from build123d import *

# Parameters (mm, degrees)
SKETCH2_R                        = 15
BOSS_EXTRUDE1_DEPTH              = 20
TAP_DRILL_FOR_M18X2_5_TAP1_D     = 15.5
TAP_DRILL_FOR_M18X2_5_TAP1_DEPTH = 15
TAP_DRILL_FOR_M18X2_5_TAP1_TIP   = 4.656669797
FILLET1_R                        = 4


with BuildPart() as part:
    # Sketch2 → Boss-Extrude1 (new body)
    with BuildSketch(Plane(origin=(0, 0, 0), x_dir=(1, 0, 0), z_dir=(0, 1, 0))):
        Circle(SKETCH2_R)
    extrude(amount=BOSS_EXTRUDE1_DEPTH)

    # Tap Drill for M18x2.5 Tap1
    with Locations(Plane(origin=(0, 0, 0), x_dir=(-1, 0, 0), z_dir=(0, -1, 0))):
        with Locations((0, 0)):
            Hole(TAP_DRILL_FOR_M18X2_5_TAP1_D / 2, depth=TAP_DRILL_FOR_M18X2_5_TAP1_DEPTH)
            with Locations((0, 0, -(TAP_DRILL_FOR_M18X2_5_TAP1_DEPTH + TAP_DRILL_FOR_M18X2_5_TAP1_TIP / 2))):  # 118° drill point
                Cone(0, TAP_DRILL_FOR_M18X2_5_TAP1_D / 2, TAP_DRILL_FOR_M18X2_5_TAP1_TIP, mode=Mode.SUBTRACT)

    # Fillet1
    fillet1_edges = [part.edges().sort_by_distance(p)[0] for p in [
        (-15, 20, 0),
    ]]
    fillet(fillet1_edges, radius=FILLET1_R)


solid = part.part
Source: CAD feature listing. Evaluate the final solid. Frame: model axes, mm. Give positions to 0.01 mm unless a question says otherwise; leave off trailing zeros. Write each loop counter-clockwise with the first axis right and the second up, starting at its lowest first coordinate (ties: lowest second). Pieces come first, ordered by that corner, then holes. Notation, with made-up numbers: (10, -24) -> (58, -24) arc R8 cw to (58, -17) -> close; hole circle Ø6 at (69, 42). An arc over 180 degrees is marked (long way). Write item = value, one per line.
Q1. First-contact query: pin 1 (1.5 mm diameter, centred on y = 14.5, z = 1.5, fed in from -X); pin 2 (1 mm diameter, centred on x = 6.5, z = 2, fed in from -Y); pin 3 (1.5 mm diameter, centred on y = 7, z = 2.5, fed in from +X). Flat tips, straight axial feed; report the tip coordinate or a pass-through.
Here are the results:
pin_1 = -14.98
pin_2 = 15.27
pin_3 = 14.9
Q2. Line query: line 1 (Z direction, x = 0, y = 5); line 2 (Z direction, x = 5.5, y = 1.75); line 3 (X direction, y = 15.25, z = 2.25). Output: solid intervals per line, ascending. Write a range as from..to.
Here are the results:
line_1 = -15..-7.75, 7.75..15
line_2 = -13.96..-5.46, 5.46..13.96
line_3 = -14.83..-6.98, 6.98..14.83
Q3. Cut plane A-A on y = 8. Return loops of the section in (x, z), then the cut area to 3 significant figures.
Here are the results:
outline = circle Ø30 at (0, 0); hole circle Ø15.5 at (0, 0)
area = 518 mm²
Q4. Mould query, pull axis Z, two halves, no side actions, for faces 1 (the face through (-14.985, 7.888, -0.66)), 2 (the face through (6, 0, 6)), 3 (the face through (-1.009, 7.605, -7.684)). Classes: +Z half, -Z half, draft (parallel to the pull), parting line (faces both ways), or undercut.
Here are the results:
face_1 = parting line
face_2 = draft
face_3 = undercut
